The listing builds one solid part. Answer for the finished solid, in the listing's coordinates (mm). A direction names the side the tool comes from. Give positions to 0.01 mm unless a question says otherwise; leave off trailing zeros. Loops run counter-clockwise (first coordinate to the right, second up) from the corner with the lowest first, then second, coordinate; pieces in that order, holes last. Notation, with made-up numbers: (75, 77) - (105, 77) arc R34 ccw to (105, 115) - close; hole circle Ø3 at (12, 85.25). An arc over 180 degrees is marked (long way). Answer in a Markdown table with one row per item. Add a question column.
```python
from build123d import *

# Parameters (mm, degrees)
F0_R     = 3
F1_DEPTH = 3
F2_DEPTH = 3
F3_R     = 2.5
F4_R     = 2.5
F5_R     = 2.5


# Not quite as in the source:
# - a feature names something its author has since deleted; it is built from what else it names


with BuildPart() as f1:
    # F0 (on Top) → F1 (new body)
    with BuildSketch(Plane.XY):
        Polygon((73.486745642, 26.9546627321), (46.6403742633, 73.8689917145), (20.8729718881, 43.5791923222), (28.6391571445, 73.9381045595), (1.4333421336, 27.2313004548), (40.5487790704, 20.0609751046), (10.3740972135, 11.6072327084), (64.4262836031, 11.3997078307), (51.0782490415, 48.8598325732), align=None)
        with Locations((37.5, 37.5)):
            Circle(F0_R, mode=Mode.SUBTRACT)
    extrude(amount=F1_DEPTH)

    # F0 (on Top) → F2 (join)
    with BuildSketch(Plane.XY):
        Polygon((73.486745642, 26.9546627321), (46.6403742633, 73.8689917145), (20.8729718881, 43.5791923222), (28.6391571445, 73.9381045595), (1.4333421336, 27.2313004548), (40.5487790704, 20.0609751046), (10.3740972135, 11.6072327084), (64.4262836031, 11.3997078307), (51.0782490415, 48.8598325732), align=None)
        with Locations((37.5, 37.5)):
            Circle(F0_R, mode=Mode.SUBTRACT)
    extrude(amount=F2_DEPTH)

    # F3
    f3_edges = [f1.edges().sort_by_distance(p)[0] for p in [
        (51.078249, 48.859833, 1.5),
    ]]
    fillet(f3_edges, radius=F3_R)

    # F4
    f4_edges = [f1.edges().sort_by_distance(p)[0] for p in [
        (20.872972, 43.579192, 1.5),
    ]]
    fillet(f4_edges, radius=F4_R)

    # F5
    f5_edges = [f1.edges().sort_by_distance(p)[0] for p in [
        (40.548779, 20.060975, 1.5),
    ]]
    fillet(f5_edges, radius=F5_R)


solid = f1.part
```
(1) A cutting plane is placed at D-D on y = 37.5. Determine the outline of the cut face in (x, z).
(2) A cutting plane is placed at B-B on z = 1.1. Determine the outline of the cut face in (x, y), plus the area to 3 significant figures.
(3) A cutting plane is placed at A-A on y = 29.5. Determine the outline of the cut face in (x, z), plus the area to 3 significant figures.
(4) Given pin 1 Ø3.5 at (x, y) = (37.5, 37.5) entering from -Z, flat-ended and moving along its own axis, determine where the tip first touches the part or whether it passes through.
(5) The mould has two halves that part along Y. Classify faces 1 (the face through (60.251, 50.083, 1.479)), 2 (the face through (37, 43, 0)), 3 (the face through (35.29, 39.53, 1.48)), 4 (the face through (20.394, 14.414, 1.479)): pulls with the +Y half, pulls with the -Y half, needs draft (parallel to the pull), parting line crosses it, or undercut.
(6) Find the intervals of material crossed by line 1 along Y through (x, z) = (37.5, 2.35); line 2 along X through (y, z) = (66, 0.6); line 3 along Y through (x, z) = (11, 1.1), in increasing order. Write a range as [from, to].
(7) A cutting plane is placed at C-C on x = 27. Determine the outline of the cut face in (y, z), plus the area to 3 significant figures.
(8) A tool of negligible diameter and unlimited length cuts with its end or side. For faces 5 (the face through (15.47, 24.66, 1.48)), 6 (the face through (59.635, 24.846, 1.479)), 7 (the face through (15.227, 50.912, 1.479)), from which of +Z, -Z, +X, -X, +Y, -Y can it reach the whole face along a straight path? Write none if from no direction.
Evaluation:
| question | item | result |
|---|---|---|
| 1 | outline | (7.41, 0) - (34.5, 0) - (34.5, 3) - (7.41, 3) - close; (40.5, 0) - (55.13, 0) - (55.13, 3) - (40.5, 3) - close; (62.7, 0) - (67.45, 0) - (67.45, 3) - (62.7, 3) - close |
| 2 | outline | (1.43, 27.23) - (29.91, 22.01) arc R2.5 cw to (30.14, 17.14) - (10.37, 11.61) - (64.43, 11.4) - (54.71, 38.67) arc R2.5 cw to (58.81, 41.3) - (73.49, 26.95) - (46.64, 73.87) - (27.88, 51.81) arc R2.5 cw to (23.55, 54.05) - (28.64, 73.94) - close; hole circle Ø6 at (37.5, 37.5) |
| 2 | area | 2,300 mm² |
| 3 | outline | (2.75, 0) - (57.98, 0) - (57.98, 3) - (2.75, 3) - close; (70.88, 0) - (72.03, 0) - (72.03, 3) - (70.88, 3) - close |
| 3 | area | 169 mm² |
| 4 | pin 1 | passes through |
| 5 | face 1 | pulls with the +Y half |
| 5 | face 2 | needs draft |
| 5 | face 3 | undercut |
| 5 | face 4 | undercut |
| 6 | line 1 | y = [11.5, 34.5], [40.5, 63.12] |
| 6 | line 2 | x = [24.02, 26.61], [39.95, 51.14] |
| 6 | line 3 | y = [11.6, 11.78], [25.48, 43.66] |
| 7 | outline | (11.54, 0) - (16.27, 0) - (16.27, 3) - (11.54, 3) - close; (22.54, 0) - (51.15, 0) - (51.15, 3) - (22.54, 3) - close; (67.53, 0) - (71.12, 0) - (71.12, 3) - (67.53, 3) - close |
| 7 | area | 111 mm² |
| 8 | face 5 | +Z, -Z, -X |
| 8 | face 6 | +Z, -Z |
| 8 | face 7 | +Z, -Z, -X, +Y |
